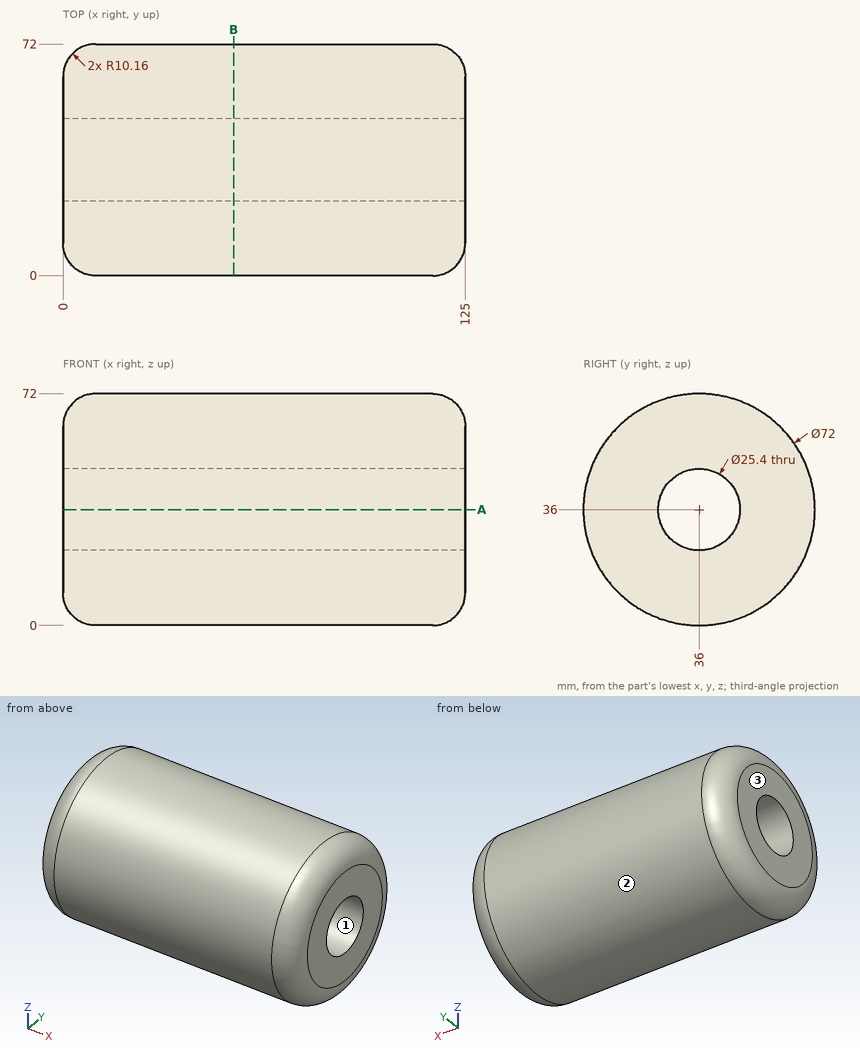
Can you work these out from the drawing? Everything is in mm from the part's minimum corner. Give positions to 0.01 mm unless a question says otherwise; leave off trailing zeros. Order: outer loops, then holes, each group sorted by start corner. A loop starts at its lowest first (then second) coordinate and runs counter-clockwise, first axis right, second up.
Item 1: If we section it at B-B, the plane x = 53: Write out the boundary of the cut face in (y, z), plus the area to 3 significant figures.
Item 2: If we section it at A-A, the plane z = 36: Write out the boundary of the cut face in (x, y), plus the area to 3 significant figures.
Item 3: I need wall thicknesses on line 1 (Z direction, x = 80, y = 36); line 2 (Z direction, x = 40, y = 38.5); line 3 (Y direction, x = 65, z = 32.5). Which ranges of each line are inside material? Lowest first, please.
Item 4: I'm going to push flat-ended pins straight in: pin 1 (6 mm diameter, centred on x = 55, z = 21.5, fed in from -Y); pin 2 (3 mm diameter, centred on x = 111, z = 9.5, fed in from +Y); pin 3 (2 mm diameter, centred on x = 42, y = 53.5, fed in from -Z). Where does each tip first touch, or does it pass through?
Item 5: If we mould it in two halves opening along Z, with no side actions, what happens to the marked faces 1, 2 and 3? For each: pulls with the +Z half, pulls with the -Z half, needs draft (parallel to the pull), parting line crosses it, or undercut.
Values:
1. outline: circle Ø72 at (36, 36); hole circle Ø25.4 at (36, 36)
1. area: 3,560 mm2
2. outline: (0, 10.16) arc R10.16 ccw to (10.16, 0) - (114.84, 0) arc R10.16 ccw to (125, 10.16) - (125, 23.3) - (0, 23.3) - close; (0, 48.7) - (125, 48.7) - (125, 61.84) arc R10.16 ccw to (114.84, 72) - (10.16, 72) arc R10.16 ccw to (0, 61.84) - close
2. area: 5,740 mm2
3. line 1: z = 0 to 23.3, 48.7 to 72
3. line 2: z = 0.09 to 23.55, 48.45 to 71.91
3. line 3: y = 0.17 to 23.79, 48.21 to 71.83
4. pin 1: stops at y = 1.89
4. pin 2: stops at y = 61.9
4. pin 3: stops at z = 4
5. face 1: undercut
5. face 2: parting line crosses it
5. face 3: needs draft
